Input: dimensioned drawing with shaded views. Units: mm. Origin: part minimum x, y, z. Give positions to 0.01 mm unless a question says otherwise; leave off trailing zeros. Order: outer loops, then holes, each group sorted by start corner. A loop starts at its lowest first (then second) coordinate and runs counter-clockwise, first axis right, second up.
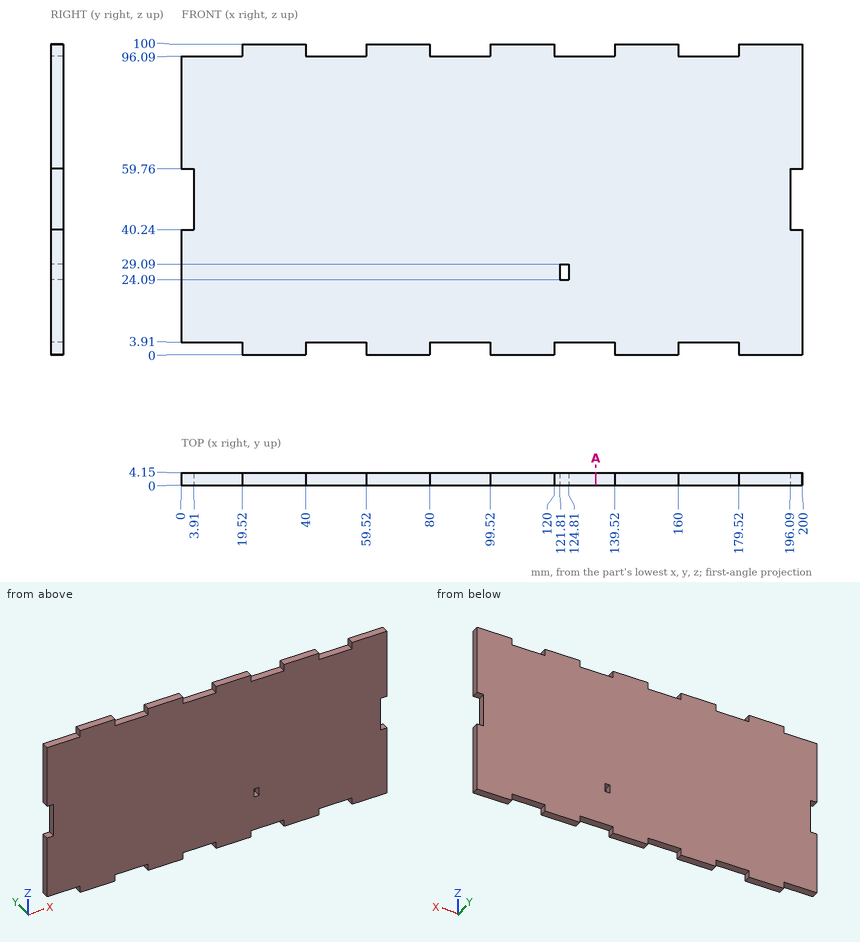
1) Cut plane A-A (x = 133.5). Return the cut outline in (y, z).
2) First-contact query: P1, Ø2, axis at y = 1, z = 2, coming from the -X side; P2, Ø2, axis at x = 125, y = 1.5, coming from the -Z side; P3, Ø2, axis at x = 125, y = 2.5, coming from the +Z side. Flat tips, straight axial feed; report the tip coordinate or a pass-through.
3) Line query: probe 1 along Z at (x, y) = (12, 0.5); probe 2 along X at (y, z) = (2.65, 27); probe 3 along X at (y, z) = (2.75, 52.5). Output: solid intervals per line, ascending.
Geometry says:
1. outline: (0, 3.91) - (4.15, 3.91) - (4.15, 96.09) - (0, 96.09) - close
2. P1: stops at x = 19.52
2. P2: stops at z = 3.91
2. P3: stops at z = 96.09
3. probe 1: z = 3.91 to 96.09
3. probe 2: x = 0 to 121.81, 124.81 to 200
3. probe 3: x = 3.91 to 196.09
